The listing builds one solid part. Answer for the finished solid, in the listing's coordinates (mm). A direction names the side the tool comes from. Give positions to 0.01 mm unless a question says otherwise; leave off trailing zeros. Write each loop counter-clockwise with the first axis right and the second up, starting at its lowest first coordinate (ties: lowest second). Pieces come first, ordered by that corner, then holes. Notation, with made-up numbers: (6.25, 1) -> (41.25, 1) arc R30 ccw to (41.25, 23) -> close; hole circle Ø9 at (64, -6). An arc over 180 degrees is marked (long way). Put each result on its own line as item: value. Start each with the question number.
1) Find the intervals of material crossed by line 1 along X through (y, z) = (-0.25, 1.25); line 2 along X through (y, z) = (-1.05, 0); line 3 along Y through (x, z) = (-6, -8.5), in increasing order. Write a range as from..to.
2) A cutting plane is placed at B-B (y = 7). Write down the section's boundary in (x, z), then the cut area to 3 significant figures.
3) A cutting plane is placed at C-C (z = 0). Give the number of separate pieces and of enclosed holes in the cut face, then the cut area to 3 significant figures.
4) For faces 5 (the cylindrical face through (-11.12, -1.143, -0.14)), 6 (the flat face through (-10.001, 11.3, 2.4)), determine the directions among +Z, -Z, +X, -X, +Y, -Y from which every point of the face is accessible in a straight line to the end or side of a thin tool.
5) For a pull along X with two mould halves and no side action, classify faces 1 (the cylindrical face through (3.78, -0.79, 1.43)), 2 (the cylindrical face through (29.43, -0.79, -9.4)), 3 (the cylindrical face through (17.93, -0.79, 0.75)), 4 (the flat face through (10, 0, 0)) as released by +X, released by -X, zero draft, split by the parting line, or undercut.
6) A cutting plane is placed at D-D (x = 13). Write down the section's boundary in (y, z), then the cut area to 3 significant figures.
7) Flat-ended cylindrical pins translate along their axes: pin 1 Ø10 at (x, z) = (4, 3) entering from +Y; pin 2 Ø5 at (y, z) = (4, -6) entering from +X. Find the tip coordinate at first contact, or state that the pin passes through.
from build123d import *

# Parameters (mm, degrees)
SKETCH1_R                  = 3
SKETCH1_R_2                = 1.5
BASE_FLANGE1_DEPTH         = 1.6
SKETCHED_START             = -30
SKETCHED_BEND1_OUTLINE_W   = 1.6
SKETCHED_BEND1_OUTLINE_H   = 20
SKETCHED_BEND1_DEPTH       = 18.399
SKETCHED_START_2           = -11.601
SKETCHED_BEND1_2_OUTLINE_R = 3
SKETCHED_BEND1_2_DEPTH     = 1.6
SKETCHED_START_3           = -11
SKETCHED_BEND1_3_DEPTH     = 22
SKETCHED_START_4           = -10
SKETCHED_BEND1_4_DEPTH     = 20


with BuildPart() as part:
    # Base-Flange1: sheet metal written as solids
    # Sketch1 → Base-Flange1 (new body)
    with BuildSketch(Plane(origin=(0, 0, 0), x_dir=(1, 0, 0), z_dir=(0, 1, 0))):
        with BuildLine():
            Line((-28, -10), (28, -10))
            ThreePointArc((28, -10), (29.414213562, -9.414213562), (30, -8))
            Line((30, -8), (30, 8))
            ThreePointArc((30, 8), (29.414213562, 9.414213562), (28, 10))
            Line((28, 10), (-28, 10))
            ThreePointArc((-28, 10), (-29.414213562, 9.414213562), (-30, 8))
            Line((-30, 8), (-30, -8))
            ThreePointArc((-30, -8), (-29.414213562, -9.414213562), (-28, -10))
        make_face()
        with Locations(Location((-20, 0, 0), (0, 0, 270))):
            Circle(SKETCH1_R, mode=Mode.SUBTRACT)
        with Locations(Location((16.666666667, 0.059373734, 0), (0, 0, 270))):
            Circle(SKETCH1_R_2, mode=Mode.SUBTRACT)
        with Locations(Location((3.333333333, 0, 0), (0, 0, 270))):
            Circle(SKETCH1_R_2, mode=Mode.SUBTRACT)
    extrude(amount=-BASE_FLANGE1_DEPTH)

    # Sketched Bend1: read off the stored shape, not the designer's step
    # Sketched Bend1 outline → Sketched Bend1 (cut)
    with BuildSketch(Plane.YZ.offset(SKETCHED_START)):
        with Locations((-0.8, 0)):
            Rectangle(SKETCHED_BEND1_OUTLINE_W, SKETCHED_BEND1_OUTLINE_H)
    extrude(amount=SKETCHED_BEND1_DEPTH, mode=Mode.SUBTRACT)

    # Sketched Bend1 2 outline → Sketched Bend1 2 (add)
    with BuildSketch(Plane.YZ.offset(SKETCHED_START_2)):
        with BuildLine():
            ThreePointArc((18.742792142, 8), (18.157005705, 9.414213563), (16.742792142, 10))
            Line((16.742792142, 10), (0, 10))
            Line((0, 10), (0, -10))
            Line((0, -10), (16.742792142, -10))
            ThreePointArc((16.742792142, -10), (18.157005705, -9.414213563), (18.742792142, -8))
            Line((18.742792142, -8), (18.742792142, 8))
        make_face()
        with Locations((8.742792142, 0)):
            Circle(SKETCHED_BEND1_2_OUTLINE_R, mode=Mode.SUBTRACT)
    extrude(amount=SKETCHED_BEND1_2_DEPTH)

    # Sketched Bend1 3 outline → Sketched Bend1 3 (cut)
    with BuildSketch(Plane.XY.offset(SKETCHED_START_3)):
        with BuildLine():
            Line((-11.601, -1.6), (-10, -1.6))
            ThreePointArc((-10, -1.6), (-11.132077957, -1.131077957), (-11.601, 0.001))
            Line((-11.601, 0.001), (-11.601, -1.6))
        make_face()
    extrude(amount=SKETCHED_BEND1_3_DEPTH, mode=Mode.SUBTRACT)

    # Sketched Bend1 4 outline → Sketched Bend1 4 (add)
    with BuildSketch(Plane.XY.offset(SKETCHED_START_4)):
        with BuildLine():
            Line((-10.001, 0), (-10, 0))
            ThreePointArc((-10, 0), (-10.000707107, 0.000292893), (-10.001, 0.001))
            Line((-10.001, 0.001), (-10.001, 0))
        make_face()
    extrude(amount=SKETCHED_BEND1_4_DEPTH)


solid = part.part
Reply:
1. line 1: x = -11.58..2.5, 4.16..15.93, 17.4..30
1. line 2: x = -11.21..1.83, 4.83..15.17, 18.17..30
1. line 3: y = -1.6..0
2. outline: (-11.6, -10) -> (-10, -10) -> (-10, -2.44) -> (-11.6, -2.44) -> close; (-11.6, 2.44) -> (-10, 2.44) -> (-10, 10) -> (-11.6, 10) -> close
2. area: 24.2 mm2
3. separate pieces: 4
3. enclosed holes: 0
3. area: 76.8 mm2
4. face 5: +Z, -Z, -X, -Y
4. face 6: +Z, -Z, +X, +Y
5. face 1: undercut
5. face 2: released by +X
5. face 3: undercut
5. face 4: zero draft
6. outline: (-1.6, -10) -> (0, -10) -> (0, 10) -> (-1.6, 10) -> close
6. area: 32.0 mm2
7. pin 1: stops at y = 0
7. pin 2: stops at x = -10
